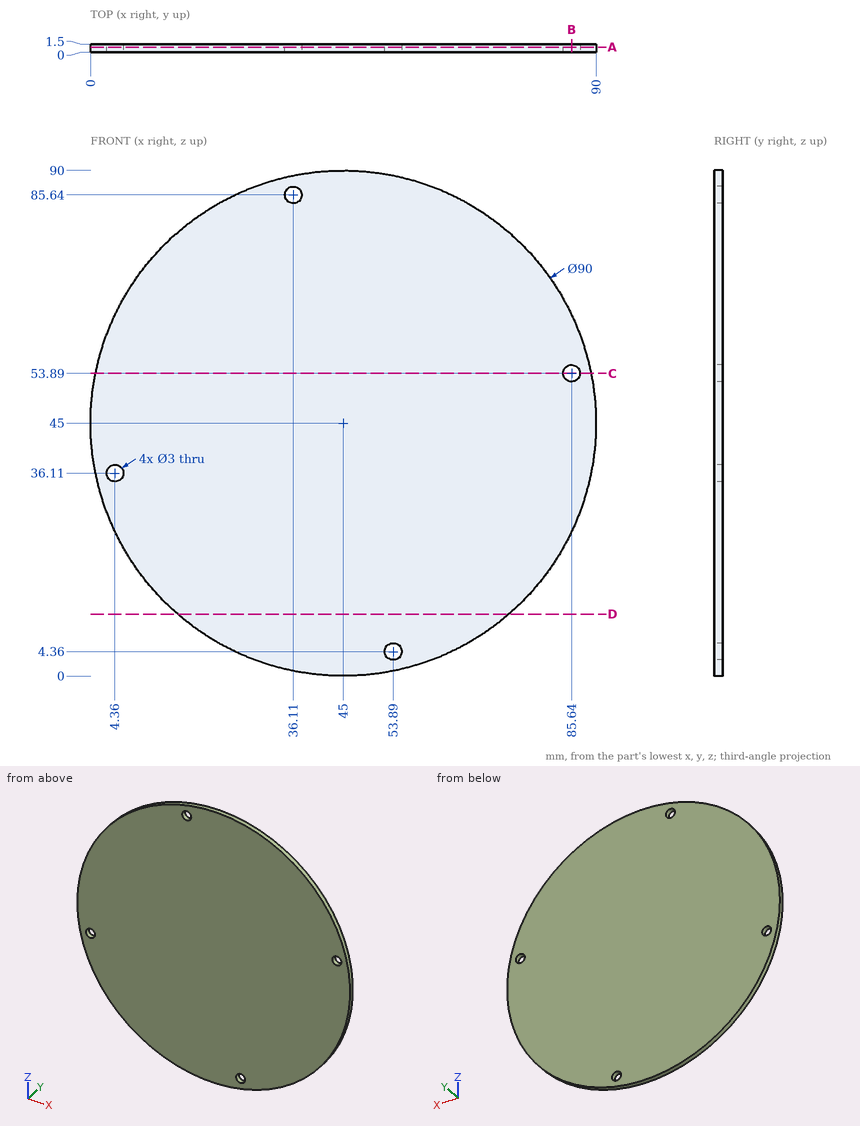
Drawing for the job (mm, zero at the part's lowest x, y, z). Round coordinates to 2 decimals unless told otherwise and drop trailing zeros. Order: outer loops, then holes, each group sorted by start corner. A loop starts at its lowest first (then second) coordinate and runs counter-clockwise, first axis right, second up. Notation, with made-up numbers: (8, 88.25) -> (44, 88.25) arc R22 ccw to (44, 105.25) -> close; hole circle Ø6 at (39.5, 57.25). An arc over 180 degrees is marked (long way). Put each result on its own line as item: value.
Q1. Band-saw the part on C-C (z = 53.89). Give the cut face in (x, y), and give its area (3 significant figures).
From the geometry:
outline: (0.89, 0) -> (84.14, 0) -> (84.14, 1.5) -> (0.89, 1.5) -> close; (87.14, 0) -> (89.11, 0) -> (89.11, 1.5) -> (87.14, 1.5) -> close
area: 128 mm2
Q2. Band-saw the part on D-D (z = 11). Give the cut face in (x, y), and give its area (3 significant figures).
From the geometry:
outline: (15.52, 0) -> (74.48, 0) -> (74.48, 1.5) -> (15.52, 1.5) -> close
area: 88.4 mm2
Q3. Wall check: line 1 (Z direction, x = 36.11, y = 0.8); line 2 (Z direction, x = 4.36, y = 1.2); line 3 (Z direction, x = 73, y = 1.4). Give the ranges that are in metal, low to high. Write a range as [from, to].
From the geometry:
line 1: z = [0.89, 84.14], [87.14, 89.11]
line 2: z = [25.68, 34.61], [37.61, 64.32]
line 3: z = [9.77, 80.23]
Q4. Band-saw the part on B-B (x = 85.64). Give the cut face in (y, z).
From the geometry:
outline: (0, 25.68) -> (1.5, 25.68) -> (1.5, 52.39) -> (0, 52.39) -> close; (0, 55.39) -> (1.5, 55.39) -> (1.5, 64.32) -> (0, 64.32) -> close
Q5. Band-saw the part on A-A (y = 0.95). Give the cut face in (x, z).
From the geometry:
outline: circle Ø90 at (45, 45); hole circle Ø3 at (4.36, 36.11); hole circle Ø3 at (36.11, 85.64); hole circle Ø3 at (53.89, 4.36); hole circle Ø3 at (85.64, 53.89)
Q6. Pin check, flat tips, straight feed: pin 1 Ø12 at (x, z) = (67.5, 38.5) entering from -Y; pin 2 Ø1.8 at (x, z) = (4.36, 36.11) entering from -Y. Stop position of each tip, or through.
From the geometry:
pin 1: stops at y = 0
pin 2: passes through
